For this review, take the finished solid that the model builds, in its own axes (mm). A direction names the side the tool comes from. Give positions to 0.01 mm unless a question says otherwise; leave off trailing zeros. Loops run counter-clockwise (first coordinate to the right, second up) from the corner with the lowest first, then second, coordinate; pieces in that order, holes last. Notation, with made-up numbers: (44.5, 41) - (60.5, 41) arc R14 ccw to (60.5, 58) - close; hole circle Ø7 at (-15.5, 0). An arc over 180 degrees is marked (long way). Use CSV: the item, a comma, the result in double quotes. Start each with the question number.
1. For faces 1 (the flat face through (-38, 7, 11)), 2 (the flat face through (-12, 1.6, 58)), 3 (the flat face through (-43, 7, 2)), 4 (the flat face through (-16.5, 7, 52)), list the 3-axis set-ups (+Z, -Z, +X, -X, +Y, -Y) from which the entire face can be reached by the end or side of a thin tool; tool diameter is ignored.
2. Mouldability with a two-part tool opening along X and no side actions: class faces 5 (the flat face through (-33, 7, 2)), 6 (the flat face through (-38, 12.6, 2)), 7 (the flat face through (-6.5, 7, 53)) as pulls with the +X half, pulls with the -X half, needs draft (parallel to the pull), parting line crosses it, or undercut.
3. Wall thickness on line 1 (X direction, y = 0.85, z = 3); line 2 (Z direction, x = -52, y = 1); line 3 (X direction, y = 3.25, z = -4): over which ranges is each line inside the solid? List them lowest first.
4. For pin 1 (1.3 mm diameter, centred on x = -26.5, y = 0.5, fed in from -Z); pin 2 (2 mm diameter, centred on y = 8, z = 2.5, fed in from -X); pin 3 (5 mm diameter, centred on x = -39, y = 6, fed in from +Z), all flat-tipped, find the tip position at first contact; note any pin that passes through.
5. Take a section at D-D on x = -35.5. Give the boundary of the cut face in (y, z), plus the area to 3 significant figures.
6. Take a section at B-B on y = 7.25. Give the boundary of the cut face in (x, z).
7. Take a section at C-C on x = -52. Give the boundary of the cut face in (y, z), plus the area to 3 significant figures.
8. Take a section at A-A on z = 52. Give the boundary of the cut face in (x, y), plus the area to 3 significant figures.
Autodesk Inventor part; units mm, degrees
ref_plane "YZ Plane" through (0, 0, 0) normal (1, 0, 0) x (0, 1, 0)
ref_plane "XZ Plane" through (0, 0, 0) normal (0, 1, 0) x (-1, 0, 0)
ref_plane "XY Plane" through (0, 0, 0) normal (0, 0, 1) x (1, 0, 0)
sketch "Sketch1" plane through (0, 0, 0) normal (0, 1, 0) x (-1, 0, 0)
  line L0 (0, 0) -> (55, 0)
  line L1 (55, 0) -> (55, 55)
  line L2 (55, 55) -> (0, 55)
  line L3 (0, 55) -> (0, 0)
  dimension "d0" = 55
  dimension "d1" = 55
extrude "Extrusion1" add sketch "Sketch1" along normal blind 1.6
sketch "Sketch2" plane through (0, 1.6, 0) normal (0, 1, 0) x (1, 0, 0)
  line L0 (-52, -52) -> (-3, -52) construction
  line L1 (-3, -52) -> (-3, -3) construction
  line L2 (-3, -3) -> (-52, -3) construction
  line L3 (-52, -3) -> (-52, -52) construction
  line L4 (-52, -52) -> (-55, -52) construction
  line L5 (-55, 0) -> (-55, -55) construction
  line L6 (-52, -52) -> (-52, -55) construction
  line L7 (-55, -55) -> (0, -55) construction
  line L8 (-3, -3) -> (-3, 0) construction
  line L9 (0, 0) -> (-55, 0) construction
  line L10 (-3, -3) -> (0, -3) construction
  line L11 (0, -55) -> (0, 0) construction
  circle A0 centre (-52, -52) radius 1.5
  circle A1 centre (-52, -3) radius 1.5
  circle A2 centre (-3, -3) radius 1.5
  circle A3 centre (-3, -52) radius 1.5
  dimension "d4" = 49
  dimension "d5" = 49
  dimension "d6" = 3
  dimension "d7" = 3
  dimension "d8" = 3
  dimension "d9" = 3
extrude "Extrusion2" cut sketch "Sketch2" against normal up to next
sketch "Sketch3" plane through (0, 1.6, 0) normal (0, 1, 0) x (1, 0, 0)
  line L0 (-6.5, -43.5) -> (-16.5, -43.5)
  line L1 (-16.5, -43.5) -> (-16.5, -61.5)
  line L2 (-16.5, -61.5) -> (-6.5, -61.5)
  line L3 (-6.5, -61.5) -> (-6.5, -43.5)
  line L4 (-55, -55) -> (0, -55)
  point P0 (0, 0)
  dimension "d12" = 10
  dimension "d13" = 18
  dimension "d14" = 6.5
  dimension "d15" = 6.5
extrude "Extrusion3" add sketch "Sketch3" along normal blind 11
sketch "Sketch4" plane through (0, 1.6, 0) normal (0, 1, 0) x (1, 0, 0)
  line L0 (-13, -11) -> (-23, -11)
  line L1 (-23, -11) -> (-23, 7)
  line L2 (-23, 7) -> (-13, 7)
  line L3 (-13, 7) -> (-13, -11)
  line L4 (-33, -11) -> (-43, -11)
  line L5 (-43, -11) -> (-43, 7)
  line L6 (-43, 7) -> (-33, 7)
  line L7 (-33, 7) -> (-33, -11)
  line L8 (0, -55) -> (0, 0)
  line L9 (0, 0) -> (-55, 0)
  dimension "d18" = 10
  dimension "d19" = 10
  dimension "d20" = 18
  dimension "d21" = 18
  dimension "d22" = 10
  dimension "d23" = 13
  dimension "d24" = 7
extrude "Extrusion4" add sketch "Sketch4" along normal blind 11
equation "\"d1\" = d0"
equation "\"d7\" = d6"
equation "\"d8\" = d6"
equation "\"d9\" = d6"
equation "\"d10\" = d5"
equation "\"d19\" = d18"
equation "\"d21\" = d20"
properties part number "Drok L298 DC Motor Driver"
Check result:
1,face 1,"+Z, +X, -X, +Y"
1,face 2,"+Z, +X, -X, -Y"
1,face 3,"+Z, -Z, -X, +Y"
1,face 4,"+Z, -X, +Y"
2,face 5,"undercut"
2,face 6,"needs draft"
2,face 7,"pulls with the +X half"
3,line 1,"x = -55 to -53.5, -50.5 to -4.5, -1.5 to 0"
3,line 2,"z = 0 to 1.5, 4.5 to 50.5, 53.5 to 55"
3,line 3,"x = -43 to -33, -23 to -13"
4,pin 1,"stops at z = 0"
4,pin 2,"stops at x = -43"
4,pin 3,"stops at z = 11"
5,outline,"(0, 0) - (1.6, 0) - (1.6, -7) - (12.6, -7) - (12.6, 11) - (1.6, 11) - (1.6, 55) - (0, 55) - close"
5,area,"286 mm²"
6,outline,"(-43, -7) - (-33, -7) - (-33, 11) - (-43, 11) - close; (-23, -7) - (-13, -7) - (-13, 11) - (-23, 11) - close; (-16.5, 43.5) - (-6.5, 43.5) - (-6.5, 61.5) - (-16.5, 61.5) - close"
7,outline,"(0, 0) - (1.6, 0) - (1.6, 1.5) - (0, 1.5) - close; (0, 4.5) - (1.6, 4.5) - (1.6, 50.5) - (0, 50.5) - close; (0, 53.5) - (1.6, 53.5) - (1.6, 55) - (0, 55) - close"
7,area,"78.4 mm²"
8,outline,"(-55, 0) - (-53.5, 0) - (-53.5, 1.6) - (-55, 1.6) - close; (-50.5, 0) - (-4.5, 0) - (-4.5, 1.6) - (-6.5, 1.6) - (-6.5, 12.6) - (-16.5, 12.6) - (-16.5, 1.6) - (-50.5, 1.6) - close; (-1.5, 0) - (0, 0) - (0, 1.6) - (-1.5, 1.6) - close"
8,area,"188 mm²"
